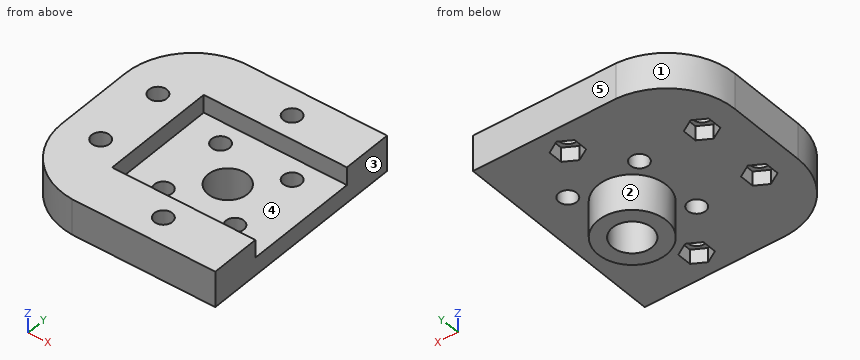
```python
from build123d import *

# Parameters (mm, degrees)
F0_W     = 40
F0_H     = 32
F0_R     = 2.5
F0_R_2   = 5.5
F1_DEPTH = 20
F2_DEPTH = 10
F3_R     = 2.5
F4_DEPTH = 4
F5_W     = 40
F5_H     = 32
F5_R     = 2.5
F5_R_2   = 9.5
F6_DEPTH = 10
F7_DEPTH = 5


with BuildPart() as f1:
    # F0 (on Top) → F1 (new body)
    with BuildSketch(Plane.XY):
        with Locations((0.5, 0)):
            Rectangle(F0_W, F0_H)
        with Locations((-10, -10)):
            Circle(F0_R, mode=Mode.SUBTRACT)
        with Locations((10, -10)):
            Circle(F0_R, mode=Mode.SUBTRACT)
        with Locations((-10, 10)):
            Circle(F0_R, mode=Mode.SUBTRACT)
        Circle(F0_R_2, mode=Mode.SUBTRACT)
        with Locations((10, 10)):
            Circle(F0_R, mode=Mode.SUBTRACT)
    extrude(amount=-F1_DEPTH)

    # F0 (on Top) → F2 (join)
    with BuildSketch(Plane.XY):
        with BuildLine():
            ThreePointArc((-19.5, 30), (-32.285489, 24.086252), (-37.5, 11))
            Line((-37.5, 11), (-37.5, -11))
            ThreePointArc((-37.5, -11), (-32.285489, -24.086252), (-19.5, -30))
            Line((-19.5, -30), (20.5, -30))
            Line((20.5, -30), (20.5, -16))
            Line((20.5, -16), (-19.5, -16))
            Line((-19.5, -16), (-19.5, 16))
            Line((-19.5, 16), (20.5, 16))
            Line((20.5, 16), (20.5, 30))
            Line((20.5, 30), (-19.5, 30))
        make_face()
        with Locations((-27.5, -10)):
            Circle(F0_R, mode=Mode.SUBTRACT)
        with Locations((0, -22.5)):
            Circle(F0_R, mode=Mode.SUBTRACT)
        with Locations((-27.5, 10)):
            Circle(F0_R, mode=Mode.SUBTRACT)
        with Locations((0, 22.5)):
            Circle(F0_R, mode=Mode.SUBTRACT)
    extrude(amount=-F2_DEPTH)

    # F3 (on face) → F4 (cut)
    with BuildSketch(Plane(origin=(0, 0, -10), x_dir=(1, 0, 0), z_dir=(0, 0, -1))):
        Polygon((3.5, 20.479274), (3.5, 24.520726), (0, 26.541452), (-3.5, 24.520726), (-3.5, 20.479274), (0, 18.458548), align=None)
        with Locations((0, 22.5)):
            Circle(F3_R, mode=Mode.SUBTRACT)
        Polygon((-24, 7.979274), (-24, 12.020726), (-27.5, 14.041452), (-31, 12.020726), (-31, 7.979274), (-27.5, 5.958548), align=None)
        with Locations((-27.5, 10)):
            Circle(F3_R, mode=Mode.SUBTRACT)
        Polygon((3.5, -24.520726), (3.5, -20.479274), (0, -18.458548), (-3.5, -20.479274), (-3.5, -24.520726), (0, -26.541452), align=None)
        with Locations((0, -22.5)):
            Circle(F3_R, mode=Mode.SUBTRACT)
        Polygon((-24, -12.020726), (-24, -7.979274), (-27.5, -5.958548), (-31, -7.979274), (-31, -12.020726), (-27.5, -14.041452), align=None)
        with Locations((-27.5, -10)):
            Circle(F3_R, mode=Mode.SUBTRACT)
    extrude(amount=-F4_DEPTH, mode=Mode.SUBTRACT)

    # F5 (on face) → F6 (cut)
    with BuildSketch(Plane(origin=(0, 0, -20), x_dir=(1, 0, 0), z_dir=(0, 0, -1))):
        with Locations((0.5, 0)):
            Rectangle(F5_W, F5_H)
        with Locations((-10, -10)):
            Circle(F5_R, mode=Mode.SUBTRACT)
        with Locations((10, -10)):
            Circle(F5_R, mode=Mode.SUBTRACT)
        Circle(F5_R_2, mode=Mode.SUBTRACT)
        with Locations((-10, 10)):
            Circle(F5_R, mode=Mode.SUBTRACT)
        with Locations((10, 10)):
            Circle(F5_R, mode=Mode.SUBTRACT)
    extrude(amount=-F6_DEPTH, mode=Mode.SUBTRACT)

    # F0 (on Top) → F7 (cut)
    with BuildSketch(Plane.XY):
        with Locations((0.5, 0)):
            Rectangle(F0_W, F0_H)
        with Locations((-10, -10)):
            Circle(F0_R, mode=Mode.SUBTRACT)
        with Locations((10, -10)):
            Circle(F0_R, mode=Mode.SUBTRACT)
        with Locations((-10, 10)):
            Circle(F0_R, mode=Mode.SUBTRACT)
        Circle(F0_R_2, mode=Mode.SUBTRACT)
        with Locations((10, 10)):
            Circle(F0_R, mode=Mode.SUBTRACT)
    extrude(amount=-F7_DEPTH, mode=Mode.SUBTRACT)


solid = f1.part
```
CAD build for the part. Positions are in the model's coordinates, mm. Face numbers are marked on the shaded views. A direction names the side the tool comes from. Round coordinates to 2 decimals unless told otherwise and drop trailing zeros. Order: outer loops, then holes, each group sorted by start corner. A loop starts at its lowest first (then second) coordinate and runs counter-clockwise, first axis right, second up.
Q1. Drop flat-ended pins along their axis: pin 1 (4 mm diameter, centred on x = -23.5, y = -17.5, fed in from -Z); pin 2 (6.5 mm diameter, centred on x = 0, y = -22.5, fed in from -Z); pin 3 (3 mm diameter, centred on x = -10.5, y = -12, fed in from +Z); pin 4 (4 mm diameter, centred on x = 10, y = -10, fed in from -Z). Give the stop position or say it passes through.
Q2. Slice it at D-D (z = -13). Write the cut outline in (x, y).
Q3. Which spindle directions (+Z, -Z, +X, -X, +Y, -Y) get a long thin tool onto all of the face, cutting with end or side? Do the marked faces 1 and 2. Say none if no direction does.
Q4. Slice it at C-C (y = 22.5). Write the cut outline in (x, z), and give its area (3 significant figures).
Q5. Slice it at B-B (z = -2.75). Write the cut outline in (x, y), and give its area (3 significant figures).
Q6. Two-plate mould, pull along Y, no slides. Class the marked faces 3, 4 and 5: pulls with the +Y half, pulls with the -Y half, needs draft (parallel to the pull), parting line crosses it, or undercut.
Q7. Wall check: L1, parallel to X at y = -10, z = -7.3; L2, parallel to X at y = -10, z = -3.05; L3, parallel to Y at x = 14.5, z = -4. Give the ranges that are in metal, low to high.
Q8. Slice it at A-A (x = -11.5). Write the cut outline in (y, z), and give its area (3 significant figures).
Results below:
1. pin 1: stops at z = -10
1. pin 2: stops at z = -6
1. pin 3: stops at z = -5
1. pin 4: passes through
2. outline: circle Ø19 at (0, 0); hole circle Ø11 at (0, 0)
3. face 1: +Z, -Z, -X, +Y
3. face 2: -Z
4. outline: (-33.63, -10) - (-3.5, -10) - (-3.5, -6) - (-2.5, -6) - (-2.5, 0) - (-33.63, 0) - close; (2.5, -6) - (3.5, -6) - (3.5, -10) - (20.5, -10) - (20.5, 0) - (2.5, 0) - close
4. area: 483 mm2
5. outline: (-37.5, -11) arc R19.03 ccw to (-19.5, -30) - (20.5, -30) - (20.5, -16) - (-19.5, -16) - (-19.5, 16) - (20.5, 16) - (20.5, 30) - (-19.5, 30) arc R19.03 ccw to (-37.5, 11) - close; hole circle Ø5 at (-27.5, -10); hole circle Ø5 at (-27.5, 10); hole circle Ø5 at (0, -22.5); hole circle Ø5 at (0, 22.5)
5. area: 1,970 mm2
6. face 3: needs draft
6. face 4: undercut
6. face 5: pulls with the +Y half
7. L1: x = -37.5 to -31, -24 to -12.5, -7.5 to 7.5, 12.5 to 20.5
7. L2: x = -37.5 to -30, -25 to -19.5
7. L3: y = -30 to -16, 16 to 30
8. outline: (-30, -10) - (-12, -10) - (-12, -5) - (-16, -5) - (-16, 0) - (-30, 0) - close; (-8, -10) - (8, -10) - (8, -5) - (-8, -5) - close; (12, -10) - (30, -10) - (30, 0) - (16, 0) - (16, -5) - (12, -5) - close
8. area: 400 mm2
